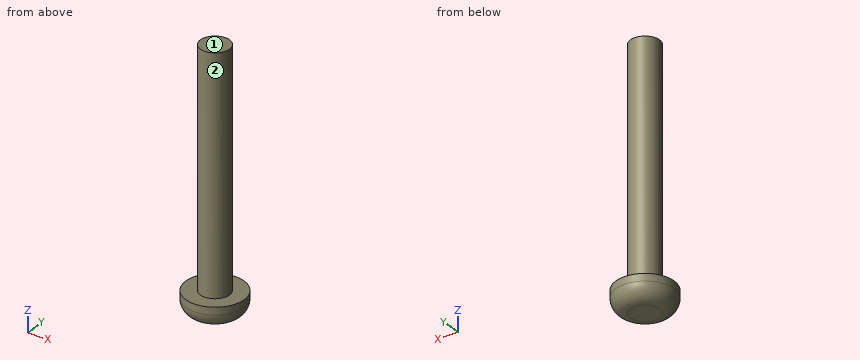
from build123d import *

# Parameters (mm, degrees)
SKETCH1_R           = 1
BOSS_EXTRUDE1_DEPTH = 16
SKETCH2_R           = 2
BOSS_EXTRUDE2_DEPTH = 1.5
FILLET1_R           = 1


with BuildPart() as part:
    # Sketch1 → Boss-Extrude1 (new body)
    with BuildSketch(Plane.XY):
        Circle(SKETCH1_R)
    extrude(amount=BOSS_EXTRUDE1_DEPTH)

    # Sketch2 → Boss-Extrude2 (add)
    with BuildSketch(Plane(origin=(0, 0, 0), x_dir=(-1, 0, 0), z_dir=(0, 0, -1))):
        Circle(SKETCH2_R)
    extrude(amount=BOSS_EXTRUDE2_DEPTH)

    # Fillet1
    fillet1_edges = [part.edges().sort_by_distance(p)[0] for p in [
        (2, 0, -1.5),
    ]]
    fillet(fillet1_edges, radius=FILLET1_R)


solid = part.part
Build history of the part. All positions in model axes, mm. Face numbers are marked on the shaded views. A direction names the side the tool comes from. Give positions to 0.01 mm unless a question says otherwise; leave off trailing zeros. Order: outer loops, then holes, each group sorted by start corner. A loop starts at its lowest first (then second) coordinate and runs counter-clockwise, first axis right, second up. Notation, with made-up numbers: M 66.25,0 L 116.25,0 A27 ccw 116.25,38 Z; hole C 34,24 d11. An arc over 180 degrees is marked long. Use one line per item in the form item = value.
1) Probe probe 1 along X at (y, z) = (-0.75, 7); probe 2 along X at (y, z) = (0.55, 5.5); probe 3 along Z at (x, y) = (0.3, -1.05). List the from-to ranges inside material, lowest first.
Calculated:
probe_1 = -0.66 to 0.66
probe_2 = -0.84 to 0.84
probe_3 = -1.5 to 0
2) Drop a flat-ended pin along its axis: pin 1 (1 mm diameter, centred on x = -0.5, y = -1, fed in from +Z). Give the stop position or say it passes through.
Calculated:
pin_1 = 16
3) Saw through at A-A (z = 13.5). Give the cut face in (x, y).
Calculated:
outline = C 0,0 d2
4) Tool access for the marked faces 1 and 2: list every direction of +Z, -Z, +X, -X, +Y, -Y with a clear straight run to the whole face (end or side of a thin tool).
Calculated:
face_1 = +Z, +X, -X, +Y, -Y
face_2 = +Z
